from build123d import *

# Parameters (mm, degrees)
PAD001_DEPTH = 5.3
FILLET_R     = 0.25
SKETCH_R     = 0.4
PAD_DEPTH    = 5


with BuildPart() as fillet_body:
    # Sketch001 → Pad001 (new body)
    with BuildSketch(Plane.XY):
        with BuildLine():
            Line((-0.9, 0.282924), (-0.9, -5.362924))
            ThreePointArc((-0.9, -5.362924), (6.99, -2.54), (-0.9, 0.282924))
        make_face()
    extrude(amount=PAD001_DEPTH)

    # Fillet
    fillet_edges = [fillet_body.edges().sort_by_distance(p)[0] for p in [
        (-0.9, -2.54, 5.3),
        (6.99, -2.54, 5.3),
    ]]
    fillet(fillet_edges, radius=FILLET_R)


with BuildPart() as diode_bridge_round_d8_9mm:
    # Sketch → Pad (new body)
    with BuildSketch(Plane.XY):
        Circle(SKETCH_R)
        with Locations((5.08, 0)):
            Circle(SKETCH_R)
        with Locations((5.08, -5.08)):
            Circle(SKETCH_R)
        with Locations((0, -5.08)):
            Circle(SKETCH_R)
    extrude(amount=-PAD_DEPTH)

    add(fillet_body.part)


solid = diode_bridge_round_d8_9mm.part
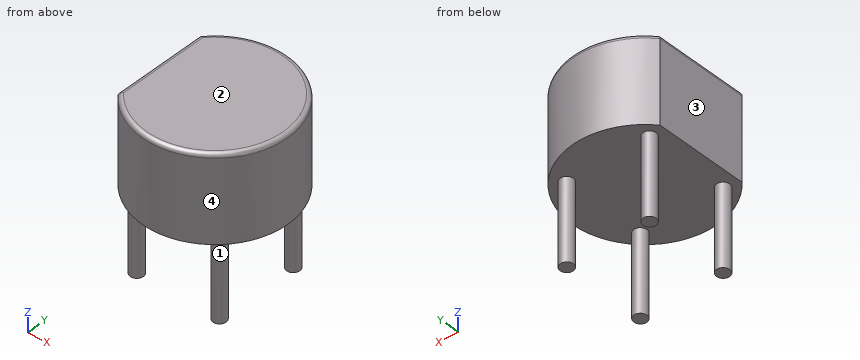
CAD build for the part. Positions are in the model's coordinates, mm. Face numbers are marked on the shaded views. Round coordinates to 2 decimals unless told otherwise and drop trailing zeros. Order: outer loops, then holes, each group sorted by start corner. A loop starts at its lowest first (then second) coordinate and runs counter-clockwise, first axis right, second up. Notation, with made-up numbers: (59, 6) - (115, 6) arc R23 ccw to (115, 40) - close; hole circle Ø7 at (-13, -7.5). An arc over 180 degrees is marked (long way). Return JSON: item names as keys, results as strings.
(1) Cut at B-B (z = -0.5). Give the cut face in (x, y), then the cut area to 3 significant figures.
Answer key:
{"outline": "circle Ø0.8 at (0, -5.08); circle Ø0.8 at (0, 0); circle Ø0.8 at (5.08, -5.08); circle Ø0.8 at (5.08, 0)", "area": "2.01 mm^2"}
(2) Cut at A-A (y = -2.54). Give the cut face in (x, z).
Answer key:
{"outline": "(-0.9, 0) - (6.99, 0) - (6.99, 5.05) arc R0.25 ccw to (6.74, 5.3) - (-0.65, 5.3) arc R0.25 ccw to (-0.9, 5.05) - close"}
(3) Pin check, flat tips, straight feed: pin 1 Ø1.5 at (x, z) = (4, -0.5) entering from +Y; pin 2 Ø1 at (x, y) = (2, -4.5) entering from -Z; pin 3 Ø1 at (y, z) = (-1.5, 2) entering from +X. Stop position of each tip, or through.
Answer key:
{"pin 1": "stops at y = 1.82", "pin 2": "stops at z = 0", "pin 3": "stops at x = 6.96"}
(4) Pull direction X, two halves, no side cores. Call the marked faces 1, 2, 3 and 4: +X half, -X half, draft (parallel to the pull), parting line (faces both ways), or undercut.
Answer key:
{"face 1": "undercut", "face 2": "draft", "face 3": "-X half", "face 4": "parting line"}
(5) Wall check: probe 1 along Y at (x, z) = (0, -1.25); probe 2 along Z at (x, y) = (2, -4); probe 3 along X at (y, z) = (-3, 1.75). Give the ranges that are in metal, low to high. Write a range as from..to.
Answer key:
{"probe 1": "y = -5.48..-4.68, -0.4..0.4", "probe 2": "z = 0..5.3", "probe 3": "x = -0.9..6.97"}
